Source: CAD feature listing. Evaluate the final solid. Frame: model axes, mm. Face numbers are marked on the shaded views. A direction names the side the tool comes from. Round coordinates to 2 decimals unless told otherwise and drop trailing zeros. Write each loop counter-clockwise with the first axis right and the second up, starting at its lowest first coordinate (ties: lowest second). Pieces come first, ordered by that corner, then holes. Notation, with made-up numbers: M 46.5,56 L 100.5,56 A7 ccw 100.5,67 Z; hole C -4.5,45 d2. An arc over 180 degrees is marked long. Answer in a Markdown table with one row per item.
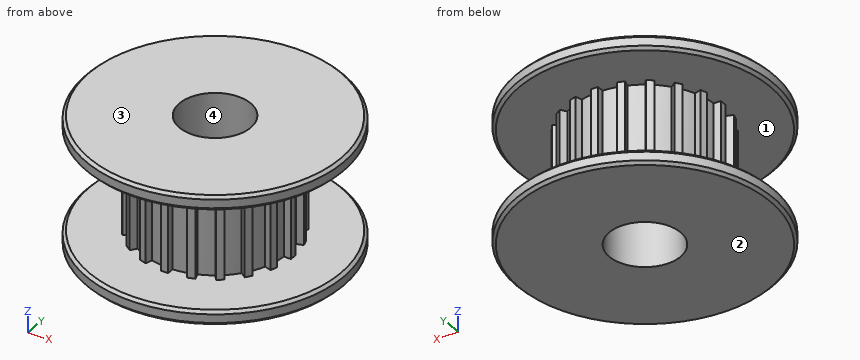
from build123d import *

# Parameters (mm, degrees)
F3_DEPTH        = 7
F3_COPIES_COUNT = 20
F4_SIZE         = 0.2


# Not quite as in the source:
# - a pattern or mirror of a feature is missing from the dataset's text; its kind, count and spacing are read off the source's solid


with BuildPart() as f1:
    # F0 (on Front) → F1 (revolve)
    with BuildSketch(Plane.XZ):
        Polygon((2.5, 9), (2.5, 0), (9, 0), (9, 1), (5, 1), (5, 8), (9, 8), (9, 9), align=None)
    revolve(axis=Axis((0, 0, 4.5), (0, 0, -1)))

    # F2 (on face) → F3 (join, through all)
    with BuildSketch(Plane.XY.offset(1)):
        with BuildLine():
            Line((-0.25, 5.4937460889), (-0.25, 4.9937460889))
            ThreePointArc((-0.25, 4.9937460889), (0, 5), (0.25, 4.9937460889))
            Line((0.25, 4.9937460889), (0.25, 5.4937460889))
            Line((0.25, 5.4937460889), (-0.25, 5.4937460889))
        make_face()
    f3 = extrude(amount=F3_DEPTH)

    # F3_copies: F3 ×20 about axis
    f3_copies_axis = Axis((0, 0, 0), (0, 0, 1))
    for i in range(1, F3_COPIES_COUNT):
        add(f3.rotate(f3_copies_axis, i * 360 / F3_COPIES_COUNT))

    # F4
    f4_edges = [f1.edges().sort_by_distance(p)[0] for p in [
        (-9, 0, 9),
        (-9, 0, 8),
        (-9, 0, 1),
        (-9, 0, 0),
    ]]
    chamfer(f4_edges, length=F4_SIZE)


solid = f1.part
Q1. Access query for the marked faces 1 and 2. Directions: +Z, -Z, +X, -X, +Y, -Y. A direction counts if a zero-diameter tool reaches every point of the face in a straight line with its end or side. Return the directions, or none.
Solutions:
| item | result |
|---|---|
| face 1 | none |
| face 2 | -Z, +X, -X, +Y, -Y |
Q2. Section A-A (x = 0). Return loops of the section in (y, z).
Solutions:
| item | result |
|---|---|
| outline | M -9,0.2 L -8.8,0 L -2.5,0 L -2.5,9 L -8.8,9 L -9,8.8 L -9,8.2 L -8.8,8 L -5.49,8 L -5.49,1 L -8.8,1 L -9,0.8 Z; M 2.5,0 L 8.8,0 L 9,0.2 L 9,0.8 L 8.8,1 L 5.49,1 L 5.49,8 L 8.8,8 L 9,8.2 L 9,8.8 L 8.8,9 L 2.5,9 Z |
Q3. Material intervals for probe 1 along Z at (x, y) = (6.75, 1); probe 2 along X at (y, z) = (4.5, 3.25); probe 3 along Y at (x, z) = (0, 4.5), sorted ascending.
Solutions:
| item | result |
|---|---|
| probe 1 | z = 0 to 1, 8 to 9 |
| probe 2 | x = -3.15 to -2.96, -2.18 to 2.18, 2.96 to 3.15 |
| probe 3 | y = -5.49 to -2.5, 2.5 to 5.49 |
Q4. Pull-direction query (Y, two-part tool) for the marked faces 3 and 4; classes: pulls with the +Y half, pulls with the -Y half, needs draft (parallel to the pull), parting line crosses it, or undercut.
Solutions:
| item | result |
|---|---|
| face 3 | needs draft |
| face 4 | undercut |
Q5. Contact query for flat-ended pins moving along their axis: pin 1 Ø0.6 at (x, z) = (0, 4) entering from -Y; pin 2 Ø0.6 at (y, z) = (0, 5.5) entering from -X; pin 3 Ø1.5 at (y, z) = (-6.5, 1.5) entering from +X. Output: stop coordinate, or through.
Solutions:
| item | result |
|---|---|
| pin 1 | stops at y = -5.49 |
| pin 2 | stops at x = -5.49 |
| pin 3 | stops at x = 6.53 |
